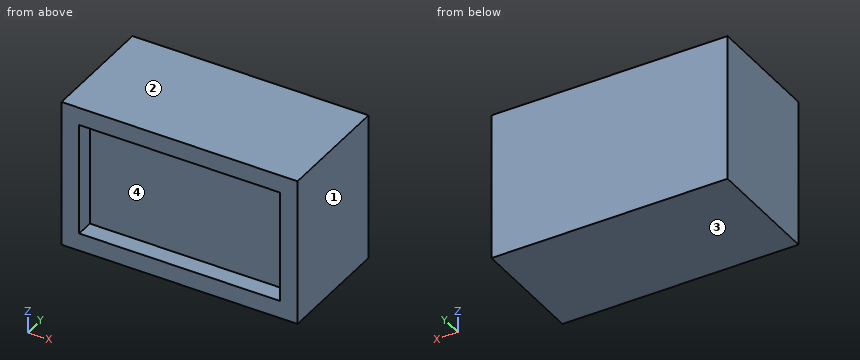
from build123d import *

# Parameters (mm, degrees)
SKETCH2_W           = 80
SKETCH2_H           = 50
BOSS_EXTRUDE1_DEPTH = 40
SKETCH3_W           = 68
SKETCH3_H           = 38
CUT_EXTRUDE1_DEPTH  = 6


with BuildPart() as part:
    # Sketch2 → Boss-Extrude1 (new body)
    with BuildSketch(Plane(origin=(0, 0, 0), x_dir=(1, 0, 0), z_dir=(0, 1, 0))):
        Rectangle(SKETCH2_W, SKETCH2_H)
    extrude(amount=BOSS_EXTRUDE1_DEPTH)

    # Sketch3 → Cut-Extrude1 (cut)
    with BuildSketch(Plane.XZ):
        Rectangle(SKETCH3_W, SKETCH3_H)
    extrude(amount=-CUT_EXTRUDE1_DEPTH, mode=Mode.SUBTRACT)


solid = part.part
Check sheet for the modelled part. Datum: model origin and axes. Units: mm. Face numbers are marked on the shaded views. Round coordinates to 2 decimals unless told otherwise and drop trailing zeros. Write each loop counter-clockwise with the first axis right and the second up, starting at its lowest first coordinate (ties: lowest second). Pieces come first, ordered by that corner, then holes. Notation, with made-up numbers: (28.25, 22) -> (32.25, 22) arc R21 cw to (32.25, 42) -> close; hole circle Ø5 at (-29.5, -11.75). An arc over 180 degrees is marked (long way). Answer as CSV lines item,"result". Start each with the question number.
1) Section check B-B on z = 8.5. Enter the section's corners in (x, y).
2) Material ranges on line 1 (Z direction, x = 21.5, y = 5); line 2 (Y direction, x = 29, z = 18), recorded low to high. Write a range as from..to.
3) Section check A-A on x = -13. Enter the section's corners in (y, z).
4) Release check for a two-part mould opening along Z. For the marked faces 1, 2, 3 and 4 record: pulls with the +Z half, pulls with the -Z half, needs draft (parallel to the pull), parting line crosses it, or undercut.
5) Go/stop test with a flat-tipped pin: P1, Ø1, axis at x = 17.5, z = 7, coming from the -Y side. Record where the tip stops, or that it passes through.
Found:
1,outline,"(-40, 0) -> (-34, 0) -> (-34, 6) -> (34, 6) -> (34, 0) -> (40, 0) -> (40, 40) -> (-40, 40) -> close"
2,line 1,"z = -25..-19, 19..25"
2,line 2,"y = 6..40"
3,outline,"(0, -25) -> (40, -25) -> (40, 25) -> (0, 25) -> (0, 19) -> (6, 19) -> (6, -19) -> (0, -19) -> close"
4,face 1,"needs draft"
4,face 2,"pulls with the +Z half"
4,face 3,"pulls with the -Z half"
4,face 4,"undercut"
5,P1,"stops at y = 6"
